from build123d import *

# Parameters (mm, degrees)
BOSS_EXTRUDE1_DEPTH = 2.54
SKETCH2_R           = 4.277185328
BOSS_EXTRUDE2_DEPTH = 2.54
BOSS_EXTRUDE3_START = 2.54
BOSS_EXTRUDE3_DEPTH = 2.54
BOSS_EXTRUDE4_START = 3.175
BOSS_EXTRUDE4_DEPTH = 1.27
BOSS_EXTRUDE5_START = -9.525
SKETCH6_R           = 0.655755768
BOSS_EXTRUDE5_DEPTH = 8.255
SKETCH7_R           = 2.759618061
BOSS_EXTRUDE6_DEPTH = 6.35
SKETCH8_R           = 0.453273613
BOSS_EXTRUDE7_DEPTH = 7.62


with BuildPart() as part:
    # Sketch1 → Boss-Extrude1 (new body)
    with BuildSketch(Plane.XY):
        with BuildLine():
            Line((0, 0), (25.4, 0))
            ThreePointArc((25.4, 0), (26.287266684, 4.829473672), (25.4, 9.658947345))
            Line((25.4, 9.658947345), (0, 9.658947345))
            ThreePointArc((0, 9.658947345), (-0.887266684, 4.829473672), (0, 0))
        make_face()
    extrude(amount=BOSS_EXTRUDE1_DEPTH)

    # Sketch2 → Boss-Extrude2 (add)
    with BuildSketch(Plane.XY.offset(2.54)):
        with Locations((12.7, 4.829473672)):
            Circle(SKETCH2_R)
    extrude(amount=BOSS_EXTRUDE2_DEPTH)

    # Sketch4 → Boss-Extrude3 (add)
    with BuildSketch(Plane.XY.offset(2.54).offset(BOSS_EXTRUDE3_START)):
        with BuildLine():
            Line((25.4, 0), (0, 0))
            ThreePointArc((0, 0), (-0.887266684, 4.829473672), (0, 9.658947345))
            Line((0, 9.658947345), (25.4, 9.658947345))
            ThreePointArc((25.4, 9.658947345), (26.287266684, 4.829473672), (25.4, 0))
        make_face()
    extrude(amount=BOSS_EXTRUDE3_DEPTH)



with BuildPart() as body_2:
    # Sketch5 → Boss-Extrude4 (new body)
    with BuildSketch(Plane.XY.offset(7.62).offset(BOSS_EXTRUDE4_START)):
        with BuildLine():
            add(Edge.make_bspline(
                [(12.7, 4.20147434), (14.810733294, 4.318694194), (18.338650019, 1.879191252), (23.539856959, 1.828704507), (24.644301026, 4.829473672)],
                knots=[0, 0, 0, 0, 0.434443821, 1, 1, 1, 1], degree=3))
            add(Edge.make_bspline(
                [(12.7, 5.457473005), (14.810733294, 5.340253151), (18.338650019, 7.779756093), (23.539856959, 7.830242837), (24.644301026, 4.829473672)],
                knots=[0, 0, 0, 0, 0.434443821, 1, 1, 1, 1], degree=3))
            add(Edge.make_bspline(
                [(12.7, 5.457473005), (10.589266706, 5.340253151), (7.061349981, 7.779756093), (1.860143041, 7.830242837), (0.755698974, 4.829473672)],
                knots=[0, 0, 0, 0, 0.434443821, 1, 1, 1, 1], degree=3))
            add(Edge.make_bspline(
                [(12.7, 4.20147434), (10.589266706, 4.318694194), (7.061349981, 1.879191252), (1.860143041, 1.828704507), (0.755698974, 4.829473672)],
                knots=[0, 0, 0, 0, 0.434443821, 1, 1, 1, 1], degree=3))
        make_face()
    extrude(amount=BOSS_EXTRUDE4_DEPTH)


with BuildPart() as part_1:
    add(part.part)

    add(body_2.part)  # Boss-Extrude5 merges body 2
    # Sketch6 → Boss-Extrude5 (add)
    with BuildSketch(Plane.XY.offset(12.065).offset(BOSS_EXTRUDE5_START)):
        with Locations((21.245716404, 4.76790511)):
            Circle(SKETCH6_R)
        with Locations((4.154283596, 4.76790511)):
            Circle(SKETCH6_R)
    extrude(amount=BOSS_EXTRUDE5_DEPTH)

    # Sketch7 → Boss-Extrude6 (add)
    with BuildSketch(Plane.XY.offset(7.62)):
        with Locations((12.7, 4.829473672)):
            Circle(SKETCH7_R)
    extrude(amount=BOSS_EXTRUDE6_DEPTH)

    # Sketch8 → Boss-Extrude7 (add)
    with BuildSketch(Plane(origin=(0, 0, 0), x_dir=(-1, 0, 0), z_dir=(0, 0, -1))):
        with Locations(Location((-12.7, 4.767836587, 0), (0, 0, 180))):
            Circle(SKETCH8_R)
    extrude(amount=BOSS_EXTRUDE7_DEPTH)


solid = part_1.part
Model file for the job. Use its own axes, mm. A direction names the side the tool comes from. Give positions to 0.01 mm unless a question says otherwise; leave off trailing zeros. Loops run counter-clockwise (first coordinate to the right, second up) from the corner with the lowest first, then second, coordinate; pieces in that order, holes last. Notation, with made-up numbers: (55.25, -32.75) -> (99.25, -32.75) arc R16 cw to (99.25, -9.75) -> close; hole circle Ø8 at (-25.75, 44.5). An arc over 180 degrees is marked (long way). Use a Markdown table: item, result. Add a question column.
(1) Mould opens along Z. For faces 4 (the flat face through (20, 5, 12.065)), 5 (the flat face through (9, 8, 2.54)), 6 (the flat face through (13, 0, 1)), 7 (the flat face through (13, 6, 0)) say: +Z half, -Z half, draft (parallel to the pull), parting line (faces both ways), or undercut.
(2) Slice it at D-D on z = 8.25. List the corners of the cut face in (x, y).
(3) Tool access for faces 1 (the flat face through (13, 0, 6)), 2 (the cylindrical face through (12.37, 4.46, -3.76)), 3 (the cylindrical face through (21.548, 4.186, 9.185)): list every direction of +Z, -Z, +X, -X, +Y, -Y with a clear straight run to the whole face (end or side of a thin tool).
(4) Wall check: line 1 along Z through (x, y) = (23, 5.75) (3 decimals); line 2 along Z through (x, y) = (6.25, 2.25); line 3 along X through (y, z) = (6.5, 12). Give the ranges that are in metal, low to high.
(5) Slice it at B-B on y = 1.25. List the corners of the cut face in (x, z), and give its area (3 significant figures).
(6) Slice it at A-A on x = 12.7. List the corners of the cut face in (y, z), and give its area (3 significant figures).
(7) Drop flat-ended pins along their axis: pin 1 Ø3 at (x, y) = (18.5, 2.5) entering from -Z; pin 2 Ø4 at (x, y) = (6, 5.5) entering from +Z (3 decimals). Give the stop position or say it passes through.
(8) Slice it at C-C on y = 3. Give the number of separate pieces and of enclosed holes in the cut face, and give its area (3 significant figures).
Filled sheet:
| question | item | result |
|---|---|---|
| 1 | face 4 | +Z half |
| 1 | face 5 | undercut |
| 1 | face 6 | draft |
| 1 | face 7 | -Z half |
| 2 | outline | circle Ø1.31 at (4.15, 4.77); circle Ø5.52 at (12.7, 4.83); circle Ø1.31 at (21.25, 4.77) |
| 3 | face 1 | +Z, -Z, +X, -X, -Y |
| 3 | face 2 | -Z |
| 3 | face 3 | none |
| 4 | line 1 | 0 to 2.54, 5.08 to 7.62, 10.795 to 12.065 |
| 4 | line 2 | 0 to 2.54, 5.08 to 7.62 |
| 4 | line 3 | 1.84 to 8.53, 10.5 to 14.9, 16.87 to 23.56 |
| 5 | outline | (-0.41, 0) -> (25.81, 0) -> (25.81, 2.54) -> (15.04, 2.54) -> (15.04, 5.08) -> (25.81, 5.08) -> (25.81, 7.62) -> (-0.41, 7.62) -> (-0.41, 5.08) -> (10.36, 5.08) -> (10.36, 2.54) -> (-0.41, 2.54) -> close |
| 5 | area | 145 mm2 |
| 6 | outline | (0, 0) -> (4.31, 0) -> (4.31, -7.62) -> (5.22, -7.62) -> (5.22, 0) -> (9.66, 0) -> (9.66, 2.54) -> (9.11, 2.54) -> (9.11, 5.08) -> (9.66, 5.08) -> (9.66, 7.62) -> (7.59, 7.62) -> (7.59, 13.97) -> (2.07, 13.97) -> (2.07, 7.62) -> (0, 7.62) -> (0, 5.08) -> (0.55, 5.08) -> (0.55, 2.54) -> (0, 2.54) -> close |
| 6 | area | 113 mm2 |
| 7 | pin 1 | z = 0 |
| 7 | pin 2 | z = 12.065 |
| 8 | separate pieces | 3 |
| 8 | enclosed holes | 0 |
| 8 | area | 198 mm2 |
